from build123d import *

# Parameters (mm, degrees)
SKETCH1_W           = 240
SKETCH1_H           = 160
BOSS_EXTRUDE2_DEPTH = 20
SKETCH5_R           = 10
CUT_EXTRUDE2_DEPTH  = 20
SKETCH6_W           = 220
SKETCH6_H           = 140
CUT_EXTRUDE3_DEPTH  = 3
SKETCH9_R           = 3
CUT_EXTRUDE4_DEPTH  = 10


with BuildPart() as part:
    # Sketch1 → Boss-Extrude2 (new body)
    with BuildSketch(Plane(origin=(0, 0, 0), x_dir=(1, 0, 0), z_dir=(0, 1, 0))):
        Rectangle(SKETCH1_W, SKETCH1_H)
    extrude(amount=BOSS_EXTRUDE2_DEPTH)

    # Sketch3 → Revolve1 (revolve)
    with BuildSketch(Plane.XY):
        Polygon((48, 20), (48, 35), (49.5, 35), (49.5, 80), (48, 80), (48, 95), (62, 95), (62, 20), align=None)
    revolve(axis=Axis((0, -30.427567953, 0), (0, 1, 0)))

    # Sketch5 → Cut-Extrude2 (cut)
    with BuildSketch(Plane.XZ):
        with Locations((95, 55)):
            Circle(SKETCH5_R)
        with Locations((-95, 55)):
            Circle(SKETCH5_R)
        with Locations((-95, -55)):
            Circle(SKETCH5_R)
        with Locations((95, -55)):
            Circle(SKETCH5_R)
    extrude(amount=-CUT_EXTRUDE2_DEPTH, mode=Mode.SUBTRACT)

    # Sketch6 → Cut-Extrude3 (cut)
    with BuildSketch(Plane.XZ):
        Rectangle(SKETCH6_W, SKETCH6_H)
    extrude(amount=-CUT_EXTRUDE3_DEPTH, mode=Mode.SUBTRACT)

    # Sketch9 → Cut-Extrude4 (cut)
    with BuildSketch(Plane(origin=(0, 20, 0), x_dir=(1, 0, 0), z_dir=(0, 1, 0))):
        with Locations((12, 0)):
            Circle(SKETCH9_R)
    extrude(amount=-CUT_EXTRUDE4_DEPTH, mode=Mode.SUBTRACT)


solid = part.part
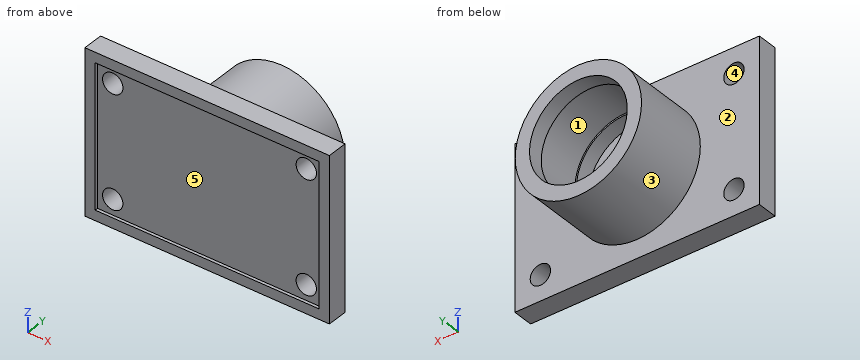
The model under review builds one solid part; all positions refer to its coordinate system, in mm. Face numbers are marked on the shaded views. A direction names the side the tool comes from. Give positions to 0.01 mm unless a question says otherwise; leave off trailing zeros. Loops run counter-clockwise (first coordinate to the right, second up) from the corner with the lowest first, then second, coordinate; pieces in that order, holes last. Notation, with made-up numbers: (-22, 34) -> (17, 34) arc R15 ccw to (17, 63) -> close; hole circle Ø7 at (8.25, 46.5). An arc over 180 degrees is marked (long way). Answer as a JSON object with one key per item and string values. Group by question number.
Q1. Wall thickness on line 1 along Z through (x, y) = (95, 16.25); line 2 along Z through (x, y) = (2, 91); line 3 along Y through (x, z) = (-18, -32.5): over which ranges is each line inside the solid? List them lowest first.
Q2. Draft analysis for pull direction Z (two halves, no side actions). For the marked faces 1, 2 and 3, state which applies: pulls with the +Z half, pulls with the -Z half, needs draft (parallel to the pull), parting line crosses it, or undercut.
Q3. Take a section at C-C (y = 39). Write out the cut boundary in (x, z).
Q4. Tool access review of the marked faces 4 and 5: name each direction out of +Z, -Z, +X, -X, +Y, -Y from which nothing blocks a thin tool from reaching the whole face with its end or side.
Q5. Take a section at B-B (x = 0). Write out the cut boundary in (y, z), plus the area to 4 significant figures.
Q6. Take a section at D-D (z = -55). Write out the cut boundary in (x, y).
Q7. Insertion check: pin 1 (6 mm diameter, centred on x = -14.5, z = 15, fed in from -Y); pin 2 (1 mm diameter, centred on x = -14.5, y = 75, fed in from +Z); pin 3 (1 mm diameter, centred on x = -43, y = 43, fed in from +Z); pin 4 (12 mm diameter, centred on x = -95, z = -55, fed in from -Y). Each pin has a flat end and moves straight along its axis. Give the tip position at first contact, or say it passes through.
Q8. Take a section at A-A (x = -95). Write out the cut boundary in (y, z), plus the area to 3 significant figures.
Answer below:
{
 "1": {"line 1": "z = -80 to -65, -45 to 45, 65 to 80", "line 2": "z = -61.97 to -47.96, 47.96 to 61.97", "line 3": "y = 3 to 20"},
 "2": {"face 1": "undercut", "face 2": "needs draft", "face 3": "parting line crosses it"},
 "3": {"outline": "circle Ø124 at (0, 0); hole circle Ø99 at (0, 0)"},
 "4": {"face 4": "+Y, -Y", "face 5": "-Y"},
 "5": {"outline": "(0, -80) -> (20, -80) -> (20, -62) -> (95, -62) -> (95, -48) -> (80, -48) -> (80, -49.5) -> (35, -49.5) -> (35, -48) -> (20, -48) -> (20, 48) -> (35, 48) -> (35, 49.5) -> (80, 49.5) -> (80, 48) -> (95, 48) -> (95, 62) -> (20, 62) -> (20, 80) -> (0, 80) -> (0, 70) -> (3, 70) -> (3, -70) -> (0, -70) -> close", "area": "4,745 mm2"},
 "6": {"outline": "(-120, 0) -> (-110, 0) -> (-110, 3) -> (-105, 3) -> (-105, 20) -> (-120, 20) -> close; (-85, 3) -> (85, 3) -> (85, 20) -> (28.62, 20) -> (28.62, 95) -> (-28.62, 95) -> (-28.62, 20) -> (-85, 20) -> close; (105, 3) -> (110, 3) -> (110, 0) -> (120, 0) -> (120, 20) -> (105, 20) -> close"},
 "7": {"pin 1": "stops at y = 3", "pin 2": "stops at z = 60.4", "pin 3": "stops at z = 45.14", "pin 4": "passes through"},
 "8": {"outline": "(0, -80) -> (20, -80) -> (20, -65) -> (3, -65) -> (3, -70) -> (0, -70) -> close; (0, 70) -> (3, 70) -> (3, 65) -> (20, 65) -> (20, 80) -> (0, 80) -> close; (3, -45) -> (20, -45) -> (20, 45) -> (3, 45) -> close", "area": "2,100 mm2"}
}
